Model file for the job. Use its own axes, mm. Round coordinates to 2 decimals unless told otherwise and drop trailing zeros. Order: outer loops, then holes, each group sorted by start corner. A loop starts at its lowest first (then second) coordinate and runs counter-clockwise, first axis right, second up. Notation, with made-up numbers: M 56,22.25 L 72,22.25 A25 ccw 72,57.25 Z; hole C 14.5,64 d10. An arc over 180 degrees is marked long. Return JSON: item names as keys, results as strings. Group by question number.
Item 1: Slice it at A-A on y = -82. Write the cut outline in (x, z).
Item 2: Probe line 1 along Y through (x, z) = (0, 2.65); line 2 along Y through (x, z) = (-18.5, 2.35); line 3 along X through (y, z) = (-19.5, 0.9). List the from-to ranges inside material, lowest first.
Item 3: Slice it at B-B on z = 2. Give the number of separate pieces and of enclosed holes in the cut face, then the cut area to 3 significant figures.
Item 4: Slice it at C-C on x = 93.5. Write the cut outline in (y, z).
Item 5: Pin check, flat tips, straight feed: pin 1 Ø2 at (x, z) = (69, 1.5) entering from +Y; pin 2 Ø1 at (y, z) = (67, 2) entering from -X; pin 3 Ø1.8 at (x, z) = (72.5, 2) entering from +Y; pin 4 Ø3.5 at (x, y) = (0, 0) entering from +Z. Stop position of each tip, or through.
Item 6: Slice it at D-D on y = -15. Write the cut outline in (x, z), then the cut area to 3 significant figures.
from build123d import *

# Parameters (mm, degrees)
SKETCH1_R           = 107.5
SKETCH1_R_2         = 2
BOSS_EXTRUDE1_DEPTH = 3.5


with BuildPart() as part:
    # Sketch1 → Boss-Extrude1 (new body)
    with BuildSketch(Plane.XY):
        Circle(SKETCH1_R)
        Circle(SKETCH1_R_2, mode=Mode.SUBTRACT)
        with BuildLine():
            Line((9, 1.5), (100, 1.5))
            ThreePointArc((100, 1.5), (101.5, 0), (100, -1.5))
            Line((100, -1.5), (9, -1.5))
            ThreePointArc((9, -1.5), (7.5, 0), (9, 1.5))
        make_face(mode=Mode.SUBTRACT)
        with BuildLine():
            Line((7.424621202, -5.303300859), (71.77133829, -69.650017947))
            ThreePointArc((71.77133829, -69.650017947), (71.77133829, -71.77133829), (69.650017947, -71.77133829))
            Line((69.650017947, -71.77133829), (5.303300859, -7.424621202))
            ThreePointArc((5.303300859, -7.424621202), (5.303300859, -5.303300859), (7.424621202, -5.303300859))
        make_face(mode=Mode.SUBTRACT)
        with BuildLine():
            Line((1.5, -9), (1.5, -100))
            ThreePointArc((1.5, -100), (0, -101.5), (-1.5, -100))
            Line((-1.5, -100), (-1.5, -9))
            ThreePointArc((-1.5, -9), (0, -7.5), (1.5, -9))
        make_face(mode=Mode.SUBTRACT)
        with BuildLine():
            Line((-5.303300859, -7.424621202), (-69.650017947, -71.77133829))
            ThreePointArc((-69.650017947, -71.77133829), (-71.77133829, -71.77133829), (-71.77133829, -69.650017947))
            Line((-71.77133829, -69.650017947), (-7.424621202, -5.303300859))
            ThreePointArc((-7.424621202, -5.303300859), (-5.303300859, -5.303300859), (-5.303300859, -7.424621202))
        make_face(mode=Mode.SUBTRACT)
        with BuildLine():
            Line((-9, -1.5), (-100, -1.5))
            ThreePointArc((-100, -1.5), (-101.5, 0), (-100, 1.5))
            Line((-100, 1.5), (-9, 1.5))
            ThreePointArc((-9, 1.5), (-7.5, 0), (-9, -1.5))
        make_face(mode=Mode.SUBTRACT)
        with BuildLine():
            Line((-7.424621202, 5.303300859), (-71.77133829, 69.650017947))
            ThreePointArc((-71.77133829, 69.650017947), (-71.77133829, 71.77133829), (-69.650017947, 71.77133829))
            Line((-69.650017947, 71.77133829), (-5.303300859, 7.424621202))
            ThreePointArc((-5.303300859, 7.424621202), (-5.303300859, 5.303300859), (-7.424621202, 5.303300859))
        make_face(mode=Mode.SUBTRACT)
        with BuildLine():
            Line((-1.5, 9), (-1.5, 100))
            ThreePointArc((-1.5, 100), (0, 101.5), (1.5, 100))
            Line((1.5, 100), (1.5, 9))
            ThreePointArc((1.5, 9), (0, 7.5), (-1.5, 9))
        make_face(mode=Mode.SUBTRACT)
        with BuildLine():
            Line((5.303300859, 7.424621202), (69.650017947, 71.77133829))
            ThreePointArc((69.650017947, 71.77133829), (71.77133829, 71.77133829), (71.77133829, 69.650017947))
            Line((71.77133829, 69.650017947), (7.424621202, 5.303300859))
            ThreePointArc((7.424621202, 5.303300859), (5.303300859, 5.303300859), (5.303300859, 7.424621202))
        make_face(mode=Mode.SUBTRACT)
    extrude(amount=BOSS_EXTRUDE1_DEPTH)


solid = part.part
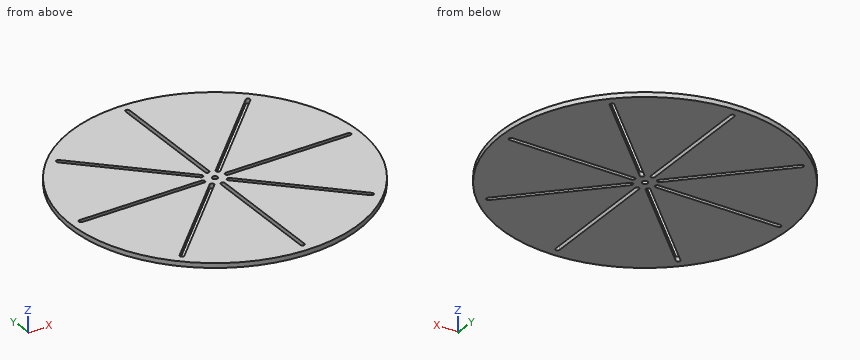
Output values:
{
 "1": {"outline": "M -69.51,0 L -1.5,0 L -1.5,3.5 L -69.51,3.5 Z; M 1.5,0 L 69.51,0 L 69.51,3.5 L 1.5,3.5 Z"},
 "2": {"line 1": "-107.5 to -101.5, -7.5 to -2, 2 to 7.5, 101.5 to 107.5", "line 2": "-105.9 to -20.62, -16.38 to -1.5, 1.5 to 16.38, 20.62 to 105.9", "line 3": "-105.72 to -21.62, -17.38 to -1.5, 1.5 to 17.38, 21.62 to 105.72"},
 "3": {"separate pieces": "1", "enclosed holes": "9", "area": "34,100 mm²"},
 "4": {"outline": "M -53.05,0 L -1.5,0 L -1.5,3.5 L -53.05,3.5 Z; M 1.5,0 L 53.05,0 L 53.05,3.5 L 1.5,3.5 Z"},
 "5": {"pin 1": "y = 83.26", "pin 2": "x = -84.46", "pin 3": "y = 80.19", "pin 4": "through"},
 "6": {"outline": "M -106.45,0 L -17.12,0 L -17.12,3.5 L -106.45,3.5 Z; M -12.88,0 L -1.5,0 L -1.5,3.5 L -12.88,3.5 Z; M 1.5,0 L 12.88,0 L 12.88,3.5 L 1.5,3.5 Z; M 17.12,0 L 106.45,0 L 106.45,3.5 L 17.12,3.5 Z", "area": "705 mm²"}
}
